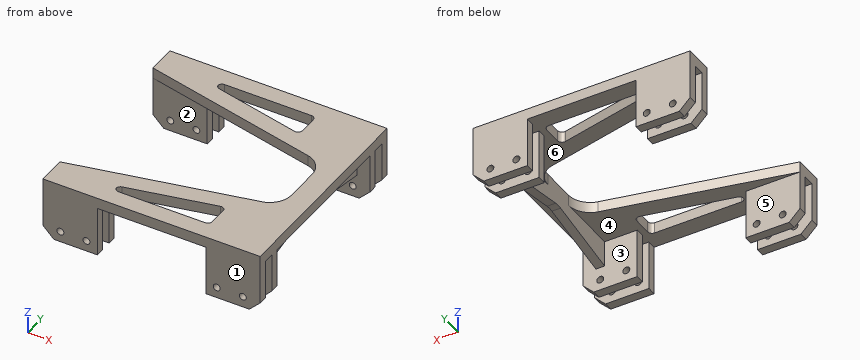
```python
from build123d import *

# Parameters (mm, degrees)
SKETCH_1_W          = 100
SKETCH_1_H          = 98.2
EXTRUDE_1_DEPTH     = 5
SKETCH_2_W          = 25
SKETCH_2_H          = 4
EXTRUDE_2_DEPTH     = 23
CHAMFER_1_SIZE      = 5
SKETCH_3_R          = 1.6
CUT_EXTRUDE_1_DEPTH = 100
SKETCH_5_W          = 90
SKETCH_5_H          = 72
CUT_EXTRUDE_2_DEPTH = 10
EXTRUDE_3_DEPTH     = 5
FILLET_1_R          = 10
EXTRUDE_4_DEPTH     = 4
CUT_EXTRUDE_3_DEPTH = 10
FILLET1_R           = 10
FILLET2_R           = 2


with BuildPart() as part:
    # 草图1 → 凸台-拉伸1 (new body)
    with BuildSketch(Plane.XY):
        with Locations((-210.886237356, -45)):
            Rectangle(SKETCH_1_W, SKETCH_1_H)
        with BuildLine():
            ThreePointArc((-245.131057565, -22.358440495), (-248.492232664, -20.607289414), (-250.886237356, -23.545446947))
            Line((-250.886237356, -23.545446947), (-250.886237356, -78))
            ThreePointArc((-250.886237356, -78), (-250.0075577, -80.121320344), (-247.886237356, -81))
            Line((-247.886237356, -81), (-224.42573361, -81))
            ThreePointArc((-224.42573361, -81), (-221.919639103, -79.649087724), (-221.670553819, -76.812993548))
            Line((-221.670553819, -76.812993548), (-245.131057565, -22.358440495))
        make_face(mode=Mode.SUBTRACT)
        with BuildLine():
            ThreePointArc((-191.655684006, -33.128922342), (-194.657829236, -31.333405344), (-197.320051564, -33.602618764))
            Line((-197.320051564, -33.602618764), (-208.123721184, -77.279649032))
            ThreePointArc((-208.123721184, -77.279649032), (-207.573803103, -79.849181859), (-205.211489311, -81))
            Line((-205.211489311, -81), (-175.458011282, -81))
            ThreePointArc((-175.458011282, -81), (-172.949810516, -79.645882413), (-172.705875596, -76.805952611))
            Line((-172.705875596, -76.805952611), (-191.655684006, -33.128922342))
        make_face(mode=Mode.SUBTRACT)
        with BuildLine():
            ThreePointArc((-176.638373042, -42.617387799), (-173.276486201, -44.360720795), (-170.886237356, -41.42334041))
            Line((-170.886237356, -41.42334041), (-170.886237356, -12))
            ThreePointArc((-170.886237356, -12), (-171.764917013, -9.878679656), (-173.886237356, -9))
            Line((-173.886237356, -9), (-186.651909841, -9))
            ThreePointArc((-186.651909841, -9), (-189.160110607, -10.354117587), (-189.404045527, -13.194047389))
            Line((-189.404045527, -13.194047389), (-176.638373042, -42.617387799))
        make_face(mode=Mode.SUBTRACT)
        with BuildLine():
            Line((-203.040454286, -12.717792993), (-213.768880163, -56.2546336))
            ThreePointArc((-213.768880163, -56.2546336), (-216.43424337, -58.526613784), (-219.43692336, -56.723847059))
            Line((-219.43692336, -56.723847059), (-238.193779397, -13.187006452))
            ThreePointArc((-238.193779397, -13.187006452), (-237.944694112, -10.350912276), (-235.438599605, -9))
            Line((-235.438599605, -9), (-205.953317692, -9))
            ThreePointArc((-205.953317692, -9), (-203.591816159, -10.149780956), (-203.040454286, -12.717792993))
        make_face(mode=Mode.SUBTRACT)
    extrude(amount=EXTRUDE_1_DEPTH)

    # 草图2 → 凸台-拉伸2 (add)
    with BuildSketch(Plane(origin=(0, 0, 0), x_dir=(-1, 0, 0), z_dir=(0, 0, -1))):
        with Locations((248.386237356, 2.1)):
            Rectangle(SKETCH_2_W, SKETCH_2_H)
        with Locations((248.386237356, -7)):
            Rectangle(SKETCH_2_W, SKETCH_2_H)
        with Locations((173.386237356, -7)):
            Rectangle(SKETCH_2_W, SKETCH_2_H)
        with Locations((173.386237356, 2.1)):
            Rectangle(SKETCH_2_W, SKETCH_2_H)
        with Locations((173.386237356, -92.1)):
            Rectangle(SKETCH_2_W, SKETCH_2_H)
        with Locations((173.386237356, -83)):
            Rectangle(SKETCH_2_W, SKETCH_2_H)
        with Locations((248.386237356, -83)):
            Rectangle(SKETCH_2_W, SKETCH_2_H)
        with Locations((248.386237356, -92.1)):
            Rectangle(SKETCH_2_W, SKETCH_2_H)
    extrude(amount=EXTRUDE_2_DEPTH)

    # 倒角1
    chamfer_1_edges = [part.edges().sort_by_distance(p)[0] for p in [
        (-160.886237356, -7, -23),
        (-160.886237356, 2.1, -23),
        (-160.886237356, -92.1, -23),
        (-160.886237356, -83, -23),
        (-260.886237356, -83, -23),
        (-260.886237356, -92.1, -23),
        (-260.886237356, 2.1, -23),
        (-260.886237356, -7, -23),
    ]]
    chamfer(chamfer_1_edges, length=CHAMFER_1_SIZE)

    # 草图3 → 切除-拉伸1 (cut)
    with BuildSketch(Plane(origin=(0, 4.1, 0), x_dir=(1, 0, 0), z_dir=(0, 1, 0))):
        with Locations(Location((-252.886237356, 18, 0), (0, 0, 270))):
            Circle(SKETCH_3_R)
        with Locations(Location((-240.886237356, 18, 0), (0, 0, 270))):
            Circle(SKETCH_3_R)
        with Locations(Location((-180.886237356, 18, 0), (0, 0, 180))):
            Circle(SKETCH_3_R)
        with Locations(Location((-168.886237356, 18, 0), (0, 0, 180))):
            Circle(SKETCH_3_R)
    extrude(amount=-CUT_EXTRUDE_1_DEPTH, mode=Mode.SUBTRACT)

    # 草图5 → 切除-拉伸2 (cut)
    with BuildSketch(Plane(origin=(0, 0, 0), x_dir=(-1, 0, 0), z_dir=(0, 0, -1))):
        with Locations((215.886237356, -45)):
            Rectangle(SKETCH_5_W, SKETCH_5_H)
    extrude(amount=-CUT_EXTRUDE_2_DEPTH, mode=Mode.SUBTRACT)

    # 草图6 → 凸台-拉伸3 (add)
    with BuildSketch(Plane(origin=(0, 0, 0), x_dir=(-1, 0, 0), z_dir=(0, 0, -1))):
        Polygon((170.886237356, -29), (260.886237356, -9), (170.886237356, -9), align=None)
        Polygon((170.886237356, -61), (170.886237356, -81), (260.886237356, -81), align=None)
    extrude(amount=-EXTRUDE_3_DEPTH)

    # 圆角1
    fillet_1_edges = [part.edges().sort_by_distance(p)[0] for p in [
        (-170.886237356, -29, 2.5),
        (-170.886237356, -61, 2.5),
    ]]
    fillet(fillet_1_edges, radius=FILLET_1_R)

    # 草图7 → 凸台-拉伸4 (add)
    with BuildSketch(Plane(origin=(-170.886237356, 0, 0), x_dir=(0, 0, -1), z_dir=(1, 0, 0))):
        Polygon((12, -9), (5, -45), (12, -81), (0, -81), (0, -9), align=None)
    extrude(amount=EXTRUDE_4_DEPTH)

    # 草图8 → 切除-拉伸3 (cut)
    with BuildSketch(Plane(origin=(0, 0, 0), x_dir=(-1, 0, 0), z_dir=(0, 0, -1))):
        Polygon((188.886237356, -16.804849371), (232.886237356, -7.027071594), (232.886237356, -3.9), (188.886237356, -3.9), align=None)
        Polygon((188.886237356, -86.1), (188.886237356, -73.195150629), (232.886237356, -82.972928406), (232.886237356, -86.1), align=None)
    extrude(amount=-CUT_EXTRUDE_3_DEPTH, mode=Mode.SUBTRACT)

    # Fillet1
    fillet1_edges = [part.edges().sort_by_distance(p)[0] for p in [
        (-168.886237356, -45, -5),
    ]]
    fillet(fillet1_edges, radius=FILLET1_R)

    # Fillet2
    # the kernel refuses this fillet: 2 mm, written as the material it adds along each edge
    with BuildSketch(Plane(origin=(-188.886237356, -16.804849371, 0), x_dir=(-0.9761870601839525, 0.2169304578186577, 0), z_dir=(0, 0, 1))) as fillet2_piece_1:
        with BuildLine():
            CenterArc((FILLET2_R * 1.24661605081, -FILLET2_R), FILLET2_R, 90, 102.528807709)
            Line((FILLET2_R * 0.270428990626, -FILLET2_R * 1.21693045782), (0, 0))
            Line((0, 0), (FILLET2_R * 1.24661605081, 0))
        make_face()
    extrude(amount=5)
    with BuildSketch(Plane(origin=(-232.886237356, -7.027071594, 0), x_dir=(0.9761870601839526, -0.21693045781865725, 0), z_dir=(0, 0, 1)), Plane(origin=(-232.886237356, -82.972928406, 0), x_dir=(0, -1, 0), z_dir=(0, 0, 1))) as fillet2_piece_2:
        with BuildLine():
            CenterArc((FILLET2_R * 0.802171606366, FILLET2_R), FILLET2_R, 192.528807709, 77.471192291)
            Line((-FILLET2_R * 0.174015453818, FILLET2_R * 0.783069542181), (0, 0))
            Line((0, 0), (FILLET2_R * 0.802171606366, 0))
        make_face()
    extrude(amount=5)
    with BuildSketch(Plane(origin=(-232.886237356, -3.9, 0), x_dir=(0, -1, 0), z_dir=(0, 0, 1)), Plane(origin=(-188.886237356, -3.9, 0), x_dir=(-1, 0, 0), z_dir=(0, 0, 1)), Plane(origin=(-232.886237356, -86.1, 0), x_dir=(1, 0, 0), z_dir=(0, 0, 1))) as fillet2_piece_3:
        with BuildLine():
            CenterArc((FILLET2_R, FILLET2_R), FILLET2_R, 180, 90)
            Line((0, FILLET2_R), (0, 0))
            Line((0, 0), (FILLET2_R, 0))
        make_face()
    extrude(amount=5)
    with BuildSketch(Plane(origin=(-188.886237356, -73.195150629, 0), x_dir=(-0.9761870601839525, -0.21693045781865739, 0), z_dir=(0, 0, 1))) as fillet2_piece_4:
        with BuildLine():
            CenterArc((FILLET2_R * 1.24661605081, FILLET2_R), FILLET2_R, 167.471192291, 102.528807709)
            Line((FILLET2_R * 0.270428990626, FILLET2_R * 1.21693045782), (0, 0))
            Line((0, 0), (FILLET2_R * 1.24661605081, 0))
        make_face()
    extrude(amount=5)
    with BuildSketch(Plane(origin=(-188.886237356, -86.1, 0), x_dir=(-1, 0, 0), z_dir=(0, 0, 1))) as fillet2_piece_5:
        with BuildLine():
            CenterArc((FILLET2_R, -FILLET2_R), FILLET2_R, 90, 90)
            Line((0, -FILLET2_R), (0, 0))
            Line((0, 0), (FILLET2_R, 0))
        make_face()
    extrude(amount=5)


solid = part.part
```
Geometry check sheet. Reference: the model listing, model coordinates, mm. Face numbers are marked on the shaded views. A direction names the side the tool comes from. Round coordinates to 2 decimals unless told otherwise and drop trailing zeros. Order: outer loops, then holes, each group sorted by start corner. A loop starts at its lowest first (then second) coordinate and runs counter-clockwise, first axis right, second up. Notation, with made-up numbers: (-13.75, 57) -> (9.25, 57) arc R8 ccw to (9.25, 72) -> close; hole circle Ø5 at (25, -9.75). An arc over 180 degrees is marked (long way). Return JSON: item names as keys, results as strings. Group by question number.
Q1. Release check for a two-part mould opening along X. For the marked faces 4, 5 and 6 record: released by +X, released by -X, zero draft, split by the parting line, or undercut.
Q2. Section check B-B, the plane z = 1.25. Record the boundary of the cut face in (x, y).
Q3. Section check C-C, the plane x = -215. Record the boundary of the cut face in (y, z).
Q4. Section check A-A, the plane z = -15.25. Count the separate pieces of the cut face and the enclosed holes in it, plus the area to 3 significant figures.
Q5. Tool access check on the marked faces 1, 2 and 3. Record the directions out of +Z, -Z, +X, -X, +Y, -Y that give a thin tool (end or side, any length) a straight path to the whole face; none if there is none.
Q6. Gauge pin test, flat ends, axial feed: pin 1 (1.5 mm diameter, centred on y = -65.5, z = -1.5, fed in from -X); pin 2 (1.5 mm diameter, centred on x = -216.5, y = -78.5, fed in from -Z); pin 3 (8 mm diameter, centred on y = -72, z = -8, fed in from +X). Record the tip position at first contact, or that the pin passes through.
Q7. Material ranges on probe 1 along Y at (x, z) = (-183, -12); probe 2 along Z at (x, y) = (-248.5, -1); probe 3 along X at (y, z) = (-56, -1.75), recorded low to high. Write a range as from..to.
Numbers:
{
 "1": {"face 4": "undercut", "face 5": "zero draft", "face 6": "undercut"},
 "2": {"outline": "(-260.89, -94.1) -> (-160.89, -94.1) -> (-160.89, 4.1) -> (-260.89, 4.1) -> (-260.89, -9) -> (-178.72, -27.26) arc R10 cw to (-170.89, -37.02) -> (-170.89, -52.98) arc R10 cw to (-178.72, -62.74) -> (-260.89, -81) -> close; hole (-232.87, -84.34) arc R2 ccw to (-230.89, -86.1) -> (-190.89, -86.1) arc R2 ccw to (-188.89, -84.1) -> (-188.89, -75.69) arc R2 ccw to (-191.32, -73.74) -> (-231.32, -82.62) arc R2 ccw to start; hole (-232.87, -5.66) arc R2 ccw to (-231.32, -7.38) -> (-191.32, -16.26) arc R2 ccw to (-188.89, -14.31) -> (-188.89, -5.9) arc R2 ccw to (-190.89, -3.9) -> (-230.89, -3.9) arc R2 ccw to start"},
 "3": {"outline": "(-94.1, 0) -> (-86.1, 0) -> (-86.1, 5) -> (-94.1, 5) -> close; (-79, 0) -> (-70.8, 0) -> (-70.8, 5) -> (-79, 5) -> close; (-19.2, 0) -> (-11, 0) -> (-11, 5) -> (-19.2, 5) -> close; (-3.9, 0) -> (4.1, 0) -> (4.1, 5) -> (-3.9, 5) -> close"},
 "4": {"separate pieces": "8", "enclosed holes": "0", "area": "800 mm^2"},
 "5": {"face 1": "+Z, -Z, +X, -X, -Y", "face 2": "-Z, -X", "face 3": "-Z"},
 "6": {"pin 1": "x = -170.89", "pin 2": "z = 0", "pin 3": "x = -166.89"},
 "7": {"probe 1": "-94.1..-90.1, -85..-81, -9..-5, 0.1..4.1", "probe 2": "0..5", "probe 3": "-170.89..-166.89"}
}
